Check sheet for the modelled part. Datum: model origin and axes. Units: mm. A direction names the side the tool comes from. Round coordinates to 2 decimals unless told otherwise and drop trailing zeros. Write each loop counter-clockwise with the first axis right and the second up, starting at its lowest first coordinate (ties: lowest second). Pieces come first, ordered by that corner, then holes. Notation, with made-up numbers: (82.5, -27.5) -> (90.5, -27.5) arc R38 ccw to (90.5, 11.5) -> close; hole circle Ø2 at (54, -30). An arc over 180 degrees is marked (long way). One line per item, written item: value.
from build123d import *

# Parameters (mm, degrees)
F1_DEPTH = 25
F2_DEPTH = 50
F0_W     = 4
F0_H     = 20.390722
F3_DEPTH = 50


with BuildPart() as f1:
    # F0 (on Right) → F1 (new body)
    with BuildSketch(Plane.YZ):
        with BuildLine():
            ThreePointArc((9.40047, 4.690722), (10.133936, 2.39615), (10.381929, 0))
            ThreePointArc((10.381929, 0), (6.955078, -8.273149), (-1.318071, -11.7))
            Line((-1.318071, -11.7), (-1.318071, -15.7))
            ThreePointArc((-1.318071, -15.7), (11.25588, -9.268728), (13.40047, 4.690722))
            Line((13.40047, 4.690722), (9.40047, 4.690722))
        make_face()
        with BuildLine():
            Line((22.40047, 4.690722), (13.40047, 4.690722))
            ThreePointArc((13.40047, 4.690722), (11.25588, -9.268728), (-1.318071, -15.7))
            Line((-1.318071, -15.7), (22.40047, -15.7))
            Line((22.40047, -15.7), (22.40047, 4.690722))
        make_face()
    extrude(amount=-F1_DEPTH)

    # F0 (on Right) → F2 (join)
    with BuildSketch(Plane.YZ):
        with BuildLine():
            Line((-1.318071, -15.7), (-1.318071, -11.7))
            ThreePointArc((-1.318071, -11.7), (-11.110197, -6.403458), (-12.036612, 4.690722))
            Line((-12.036612, 4.690722), (-16.036612, 4.690722))
            ThreePointArc((-16.036612, 4.690722), (-13.892023, -9.268728), (-1.318071, -15.7))
        make_face()
    extrude(amount=-F2_DEPTH)

    # F0 (on Right) → F3 (join)
    with BuildSketch(Plane.YZ):
        with Locations((24.40047, -5.504639)):
            Rectangle(F0_W, F0_H)
    extrude(amount=-F3_DEPTH)


with BuildPart() as f4_1:
    # F4: copy of F1
    add(f1.part)


with BuildPart() as f5_1:
    # F5: instance of F4_1
    add(f4_1.part.mirror(Plane(origin=(0, 10.566171, -6.716884), x_dir=(0, 1, 0), z_dir=(1, 0, 0))))


solid = f1.part
Item 1: Sectioned sample at D-D (z = 1). Enter the section's corners in (x, y), then the cut area to 3 significant figures.
Result set:
outline: (-50, -16.78) -> (0, -16.78) -> (0, -12.98) -> (-50, -12.98) -> close; (-50, 22.4) -> (-25, 22.4) -> (-25, 10.34) -> (0, 10.34) -> (0, 26.4) -> (-50, 26.4) -> close
area: 692 mm^2
Item 2: Sectioned sample at C-C (x = -11.5). Enter the section's corners in (y, z).
Result set:
outline: (-16.04, 4.69) arc R15.51 ccw to (-1.32, -15.7) -> (26.4, -15.7) -> (26.4, 4.69) -> (9.4, 4.69) arc R11.7 cw to (10.38, 0) arc R11.7 cw to (-1.32, -11.7) arc R11.7 cw to (-12.04, 4.69) -> close
Item 3: Sectioned sample at B-B (z = -5.5). Enter the section's corners in (x, y).
Result set:
outline: (-50, -15.89) -> (0, -15.89) -> (0, -11.64) -> (-50, -11.64) -> close; (-50, 22.4) -> (-25, 22.4) -> (-25, 9.01) -> (0, 9.01) -> (0, 26.4) -> (-50, 26.4) -> close
Item 4: Release check for a two-part mould opening along Y. For faces 3 (the flat face through (-25, 13, -8)), 4 (the flat face through (-25, 26.4, -6)), 5 (the cylindrical face through (-24.65, -14.01, -9.1)) record: pulls with the +Y half, pulls with the -Y half, needs draft (parallel to the pull), parting line crosses it, or undercut.
Result set:
face 3: undercut
face 4: pulls with the +Y half
face 5: pulls with the -Y half
Item 5: Tool access check on faces 1 (the flat face through (-14, 12, -15.7)), 2 (the flat face through (-37, 22.4, -6)). Record the directions out of +Z, -Z, +X, -X, +Y, -Y that give a thin tool (end or side, any length) a straight path to the whole face; none if there is none.
Result set:
face 1: -Z, +X, -X, +Y, -Y
face 2: +Z, -Z, -X
Item 6: Material ranges on line 1 along X through (y, z) = (12.5, 3.5); line 2 along Y through (x, z) = (-7, 0.25); line 3 along Y through (x, z) = (-42.5, -3.75), recorded low to high.
Result set:
line 1: -25 to 0
line 2: -16.82 to -13.02, 10.38 to 26.4
line 3: -16.41 to -12.4, 22.4 to 26.4
Item 7: Depth check by flat-ended pin: pin 1 (1 mm diameter, centred on x = -17, y = -2.5, fed in from -Z) (3 decimals); pin 2 (1.5 mm diameter, centred on x = -35, z = -11, fed in from -Y); pin 3 (6 mm diameter, centred on x = -36, z = -8.5, fed in from -Y). Enter the tip coordinate at first touch or a pass-through.
Result set:
pin 1: z = -15.685
pin 2: y = -13.12
pin 3: y = -15.89
Item 8: Sectioned sample at A-A (x = -40). Enter the section's corners in (y, z).
Result set:
outline: (-16.04, 4.69) arc R15.51 ccw to (-1.32, -15.7) -> (-1.32, -11.7) arc R11.7 cw to (-12.04, 4.69) -> close; (22.4, -15.7) -> (26.4, -15.7) -> (26.4, 4.69) -> (22.4, 4.69) -> close
